```python
from build123d import *

# Parameters (mm, degrees)
SKETCH_1_W          = 49.2
SKETCH_1_H          = 30
EXTRUDE_1_DEPTH     = 22
SKETCH_2_W          = 49.2
SKETCH_2_H          = 2
EXTRUDE_2_DEPTH     = 20
CUT_EXTRUDE_1_DEPTH = 7
SKETCH_4_W          = 20
SKETCH_4_H          = 18
CUT_EXTRUDE_2_DEPTH = 50
SKETCH_5_R          = 2
CUT_EXTRUDE_3_DEPTH = 22
SKETCH_7_W          = 15
SKETCH_7_H          = 8
CUT_EXTRUDE_4_DEPTH = 2


with BuildPart() as part:
    # 스케치1 → 보스-돌출1 (new body)
    with BuildSketch(Plane(origin=(0, 0, 0), x_dir=(1, 0, 0), z_dir=(0, 1, 0))):
        with Locations((0.975657895, 5.148026316)):
            Rectangle(SKETCH_1_W, SKETCH_1_H)
    extrude(amount=EXTRUDE_1_DEPTH)

    # 스케치2 → 보스-돌출2 (add)
    with BuildSketch(Plane(origin=(0, 22, 0), x_dir=(1, 0, 0), z_dir=(0, 1, 0))):
        with Locations((0.975657895, 19.148026316)):
            Rectangle(SKETCH_2_W, SKETCH_2_H)
        with Locations((0.975657895, 14.148026316)):
            Rectangle(SKETCH_2_W, SKETCH_2_H)
    extrude(amount=EXTRUDE_2_DEPTH)

    # 스케치3 → 컷-돌출1 (cut)
    with BuildSketch(Plane(origin=(0, 0, -20.148026316), x_dir=(-1, 0, 0), z_dir=(0, 0, -1))):
        with BuildLine():
            Line((-25.575657895, 42), (23.624342105, 42))
            Line((23.624342105, 42), (23.624342105, 34.364931606))
            ThreePointArc((23.624342105, 34.364931606), (-0.983636552, 32.000665788), (-25.575657895, 34.525512861))
            Line((-25.575657895, 34.525512861), (-25.575657895, 42))
        make_face()
    extrude(amount=-CUT_EXTRUDE_1_DEPTH, mode=Mode.SUBTRACT)

    # 스케치4 → 컷-돌출2 (cut)
    with BuildSketch(Plane.ZY.offset(23.624342105)):
        with Locations((-0.148026316, 11)):
            Rectangle(SKETCH_4_W, SKETCH_4_H)
    extrude(amount=-CUT_EXTRUDE_2_DEPTH, mode=Mode.SUBTRACT)

    # 스케치5 → 컷-돌출3 (cut)
    with BuildSketch(Plane.XZ):
        with Locations((13.675657895, 5.851973684)):
            Circle(SKETCH_5_R)
        with Locations((-11.724342105, 5.851973684)):
            Circle(SKETCH_5_R)
    extrude(amount=-CUT_EXTRUDE_3_DEPTH, mode=Mode.SUBTRACT)

    # 스케치7 → 컷-돌출4 (cut)
    with BuildSketch(Plane(origin=(0, 22, 0), x_dir=(1, 0, 0), z_dir=(0, 1, 0))):
        with Locations((1.075657895, 6.148026316)):
            Rectangle(SKETCH_7_W, SKETCH_7_H)
    extrude(amount=-CUT_EXTRUDE_4_DEPTH, mode=Mode.SUBTRACT)


solid = part.part
```
Input: part model. Units: mm. Frame: model coordinates. A direction names the side the tool comes from. Give positions to 0.01 mm unless a question says otherwise; leave off trailing zeros. Order: outer loops, then holes, each group sorted by start corner. A loop starts at its lowest first (then second) coordinate and runs counter-clockwise, first axis right, second up. Notation, with made-up numbers: M -11.5,75 L 13.5,75 A30 ccw 13.5,113 Z; hole C -9,-13 d7. An arc over 180 degrees is marked long. Return JSON: item names as keys, results as strings.
Item 1: Ray query, probe 1 along Y at (x, z) = (-10, -9); probe 2 along Z at (x, y) = (3.5, 24.5); probe 3 along Y at (x, z) = (-5, -17.75). Return the intervals inside material, ascending.
Solutions:
{"probe 1": "0 to 2, 20 to 22", "probe 2": "-20.15 to -18.15, -15.15 to -13.15", "probe 3": "0 to 22"}
Item 2: Cut plane D-D (x = 5). Return loops of the section in (y, z).
Solutions:
{"outline": "M 0,-20.15 L 32.08,-20.15 L 32.08,-18.15 L 22,-18.15 L 22,-15.15 L 32.08,-15.15 L 32.08,-13.15 L 22,-13.15 L 22,-10.15 L 2,-10.15 L 2,9.85 L 0,9.85 Z; M 20,-2.15 L 22,-2.15 L 22,9.85 L 20,9.85 Z"}
Item 3: Access query for faces 1 (the flat face through (1, 27, -13.148)), 2 (the flat face through (1, 2, 0)), 3 (the flat face through (1, 27, -15.148)). Directions: +Z, -Z, +X, -X, +Y, -Y. A direction counts if a zero-diameter tool reaches every point of the face in a straight line with its end or side. Return the directions, or none.
Solutions:
{"face 1": "+Z, +X, -X, +Y", "face 2": "+Z, +X, -X", "face 3": "+X, -X, +Y"}
Item 4: Cut plane A-A (z = -4.5). Return loops of the section in (x, y), then the cut area to 3 significant figures.
Solutions:
{"outline": "M -23.62,0 L 25.58,0 L 25.58,2 L -23.62,2 Z; M -23.62,20 L -6.42,20 L -6.42,22 L -23.62,22 Z; M 8.58,20 L 25.58,20 L 25.58,22 L 8.58,22 Z", "area": "167 mm^2"}
Item 5: Cut plane C-C (x = 13). Return loops of the section in (y, z), then the cut area to 3 significant figures.
Solutions:
{"outline": "M 0,-20.15 L 32.62,-20.15 L 32.62,-18.15 L 22,-18.15 L 22,-15.15 L 32.62,-15.15 L 32.62,-13.15 L 22,-13.15 L 22,3.97 L 20,3.97 L 20,-10.15 L 2,-10.15 L 2,3.97 L 0,3.97 Z; M 0,7.73 L 2,7.73 L 2,9.85 L 0,9.85 Z; M 20,7.73 L 22,7.73 L 22,9.85 L 20,9.85 Z", "area": "327 mm^2"}
Item 6: Cut plane B-B (z = -1). Return loops of the section in (x, y), then the cut area to 3 significant figures.
Solutions:
{"outline": "M -23.62,0 L 25.58,0 L 25.58,2 L -23.62,2 Z; M -23.62,20 L 25.58,20 L 25.58,22 L -23.62,22 Z", "area": "197 mm^2"}
Item 7: First-contact query: P1, Ø1, axis at x = 1, y = 13.5, coming from the +Z side; P2, Ø4.5, axis at x = 13.68, z = 5.85, coming from the +Y side; P3, Ø3, axis at x = -11.72, z = 5.85, coming from the +Y side; P4, Ø6.5, axis at x = -0.5, y = 26, coming from the +Z side. Flat tips, straight axial feed; report the tip coordinate or a pass-through.
Solutions:
{"P1": "z = -10.15", "P2": "y = 22", "P3": "through", "P4": "z = -13.15"}
Item 8: Pull-direction query (Z, two-part tool) for faces 4 (the flat face through (1, 1, 9.852)), 5 (the cylindrical face through (-13.722, 20.986, 5.94)), 6 (the cylindrical face through (1, 32, -14)); classes: +Z half, -Z half, draft (parallel to the pull), parting line (faces both ways), or undercut.
Solutions:
{"face 4": "+Z half", "face 5": "undercut", "face 6": "draft"}
